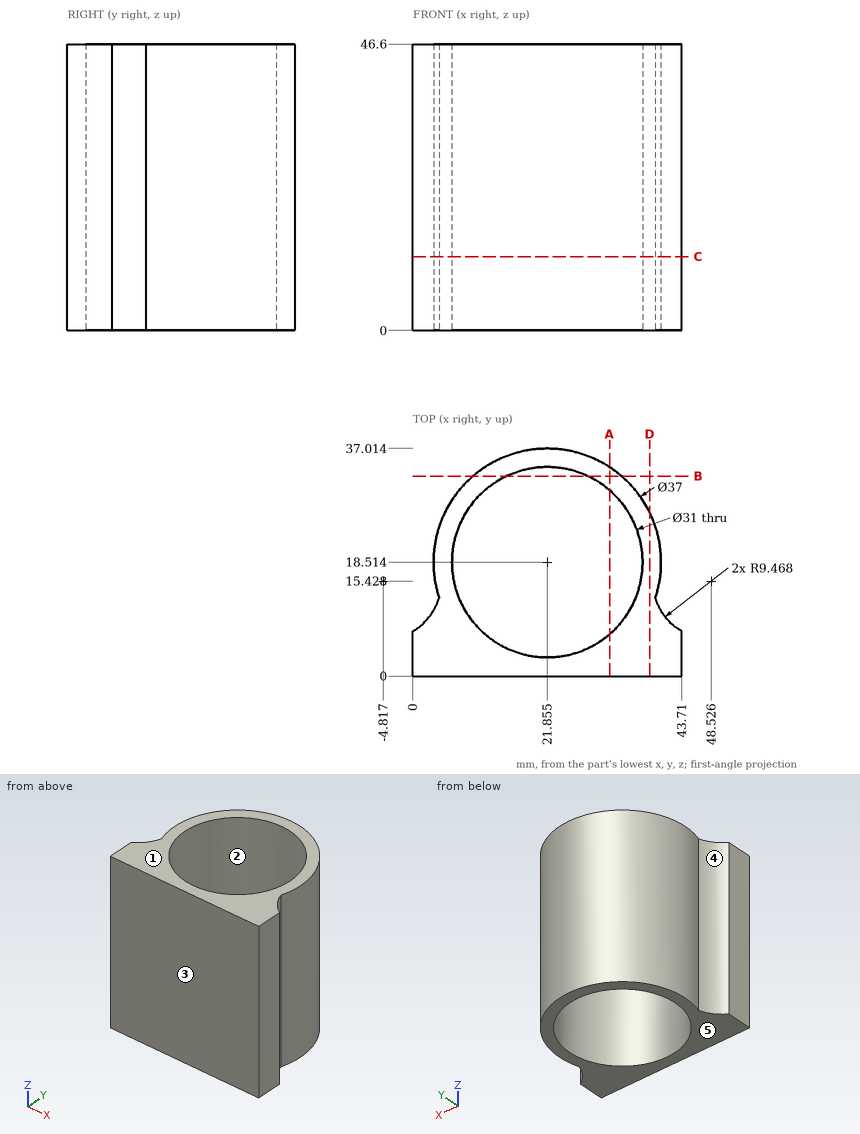
The drawing under review shows one solid part. Ordinate dimensions are in mm from its lowest x, y, z. A direction names the side the tool comes from. Coordinates: 2 decimals unless noted, no trailing zeros. Write each loop counter-clockwise with the first axis right and the second up, starting at its lowest first coordinate (ties: lowest second). Pieces come first, ordered by that corner, then holes. Notation, with made-up numbers: (-18, 55.25) - (6, 55.25) arc R17 ccw to (6, 86.25) - close; hole circle Ø8 at (65, -21). An arc over 180 degrees is marked (long way). Use one line per item in the form item = value.
Q1. Machinability: for the marked faces 4 and 5, which of the approach directions +Z, -Z, +X, -X, +Y, -Y give a long, thin tool a straight path to every point of the face, cutting with its end or side? Answer none if there is none.
Taken from the geometry:
face_4 = +Z, -Z, -X
face_5 = -Z, +X, -X, +Y, -Y
Q2. The part is to be moulded in two halves that separate along Y. For the marked faces 1, 2 and 3, say which applies: +Y half, -Y half, draft (parallel to the pull), parting line (faces both ways), or undercut.
Taken from the geometry:
face_1 = draft
face_2 = undercut
face_3 = -Y half
Q3. Consider section D-D (x = 38.5). Write out the cut boundary in (y, z).
Taken from the geometry:
outline = (0, 0) - (26.59, 0) - (26.59, 46.6) - (0, 46.6) - close
Q4. Consider section A-A (x = 32). Write out the cut boundary in (y, z) (1 decimal).
Taken from the geometry:
outline = (0, 0) - (6.8, 0) - (6.8, 46.6) - (0, 46.6) - close; (30.2, 0) - (34, 0) - (34, 46.6) - (30.2, 46.6) - close
Q5. For probe 1 along X at (y, z) = (19, 20.5); probe 2 along X at (y, z) = (25, 16); probe 3 along Y at (x, z) = (31, 28) (1 decimal), list the stretches that pass through material, from the lowest coordinate up.
Taken from the geometry:
probe_1 = 3.36 to 6.36, 37.35 to 40.35
probe_2 = 4.53 to 7.78, 35.93 to 39.18
probe_3 = 0 to 6, 31 to 34.6
Q6. Consider section C-C (z = 12). Write out the cut boundary in (x, y) (1 decimal).
Taken from the geometry:
outline = (0, 0) - (43.7, 0) - (43.7, 7.3) arc R9.5 cw to (39.4, 12.8) arc R18.5 ccw (long way) to (4.3, 12.8) arc R9.5 cw to (0, 7.3) - close; hole circle Ø31 at (21.9, 18.5)
Q7. Insertion check: pin 1 Ø1.5 at (x, z) = (10.5, 31) entering from +Y; pin 2 Ø1.5 at (x, z) = (13.5, 13) entering from +Y; pin 3 Ø18.5 at (x, y) = (21.85, 18.51) entering from -Z; pin 4 Ø4 at (x, z) = (25, 14.5) entering from +Y. Each pin has a flat end and moves straight along its axis. Give the tip position at first contact, or say it passes through.
Taken from the geometry:
pin_1 = 33.67
pin_2 = 35.38
pin_3 = through
pin_4 = 36.98
Q8. Consider section B-B (y = 32.5). Write out the cut boundary in (x, z) (1 decimal).
Taken from the geometry:
outline = (9.7, 0) - (15.2, 0) - (15.2, 46.6) - (9.7, 46.6) - close; (28.5, 0) - (34, 0) - (34, 46.6) - (28.5, 46.6) - close
